Job drawing, mm, ordinate dimensions from the low corner. One solid piece. A direction names the side the tool comes from. Round coordinates to 2 decimals unless told otherwise and drop trailing zeros. Order: outer loops, then holes, each group sorted by start corner. A loop starts at its lowest first (then second) coordinate and runs counter-clockwise, first axis right, second up. Notation, with made-up numbers: (-37.75, -23) -> (-28.75, -23) arc R37 ccw to (-28.75, 15) -> close; hole circle Ø2 at (22, -30). An arc over 180 degrees is marked (long way). Return JSON: item names as keys, results as strings. Group by question number.
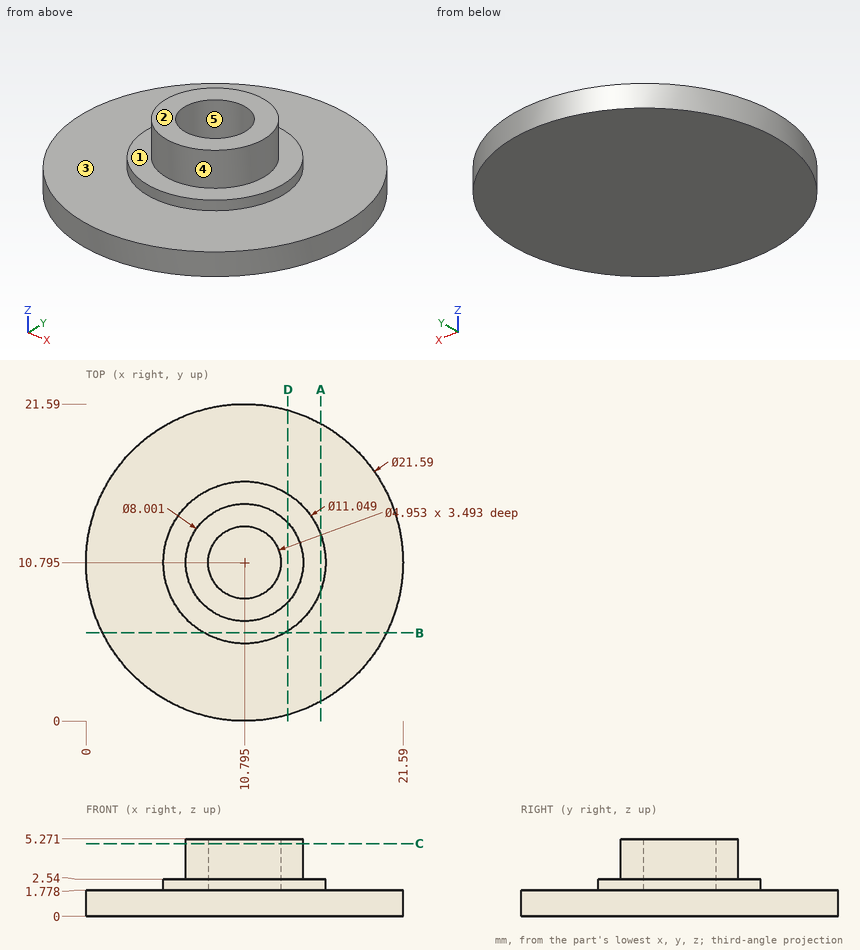
(1) Saw through at C-C, the plane z = 4.95. List the corners of the cut face in (x, y) (1 decimal).
(2) Saw through at B-B, the plane y = 6. List the corners of the cut face in (x, z).
(3) Saw through at D-D, the plane x = 13.75. List the corners of the cut face in (y, z).
(4) Mould opens along X. For the marked faces 3, 4 and 5 say: pulls with the +X half, pulls with the -X half, needs draft (parallel to the pull), parting line crosses it, or undercut.
(5) Pin check, flat tips, straight feed: P1, Ø3, axis at x = 9, y = 10.5, coming from the -Z side; P2, Ø2, axis at x = 8.5, z = 3, coming from the -Y side. Stop position of each tip, or through.
(6) Saw through at A-A, the plane x = 16. List the corners of the cut face in (y, z).
(7) Probe L1, parallel to Z at x = 18, y = 13; L2, parallel to Z at x = 7, y = 13; L3, parallel to Y at x = 11.5, z = 5. List the from-to ranges inside material, lowest first. Write a range as [from, to].
(8) Tool access for the marked faces 1 and 2: list every direction of +Z, -Z, +X, -X, +Y, -Y with a clear straight run to the whole face (end or side of a thin tool).
Results are:
{
 "1": {"outline": "circle Ø8 at (10.8, 10.8); hole circle Ø5 at (10.8, 10.8)"},
 "2": {"outline": "(1.12, 0) -> (20.47, 0) -> (20.47, 1.78) -> (13.54, 1.78) -> (13.54, 2.54) -> (8.05, 2.54) -> (8.05, 1.78) -> (1.12, 1.78) -> close"},
 "3": {"outline": "(0.41, 0) -> (21.18, 0) -> (21.18, 1.78) -> (15.46, 1.78) -> (15.46, 2.54) -> (13.49, 2.54) -> (13.49, 5.27) -> (8.1, 5.27) -> (8.1, 2.54) -> (6.13, 2.54) -> (6.13, 1.78) -> (0.41, 1.78) -> close"},
 "4": {"face 3": "needs draft", "face 4": "parting line crosses it", "face 5": "undercut"},
 "5": {"P1": "stops at z = 0", "P2": "stops at y = 5.45"},
 "6": {"outline": "(1.34, 0) -> (20.25, 0) -> (20.25, 1.78) -> (12.65, 1.78) -> (12.65, 2.54) -> (8.94, 2.54) -> (8.94, 1.78) -> (1.34, 1.78) -> close"},
 "7": {"L1": "z = [0, 1.78]", "L2": "z = [0, 2.54]", "L3": "y = [6.86, 8.42], [13.17, 14.73]"},
 "8": {"face 1": "+Z", "face 2": "+Z, +X, -X, +Y, -Y"}
}
